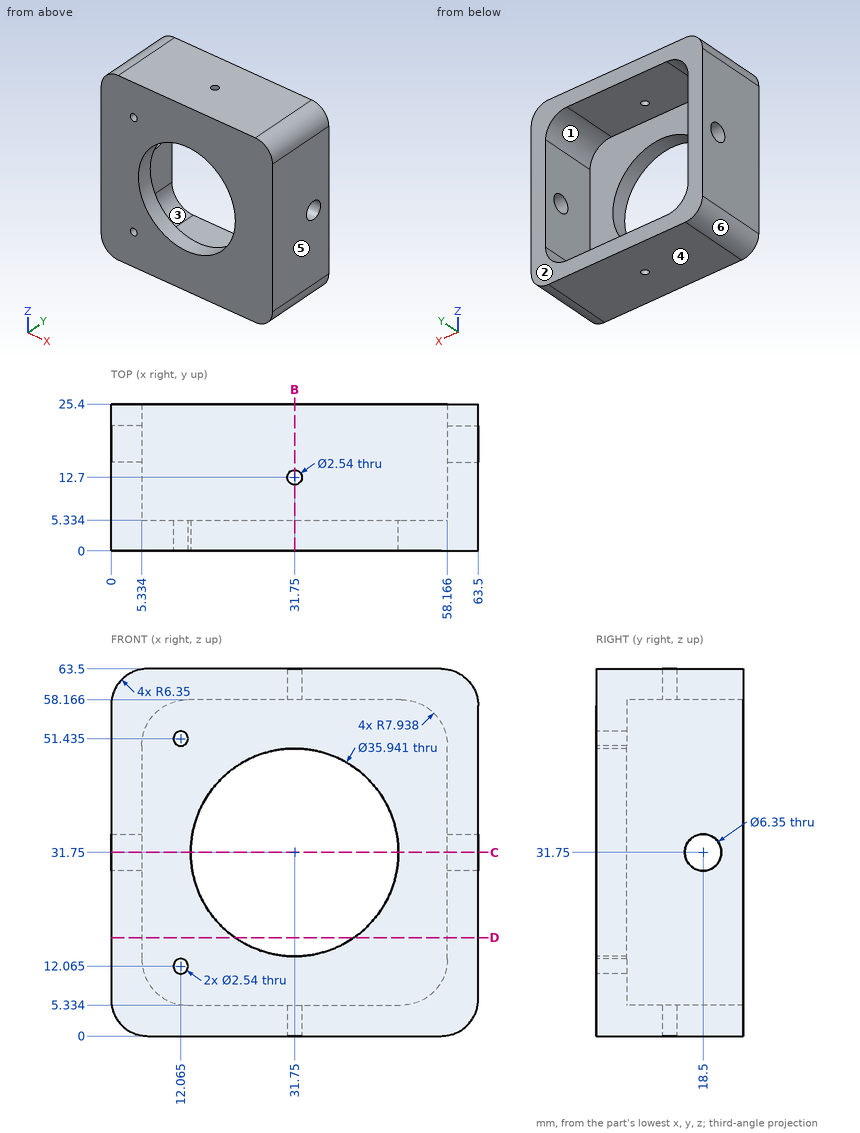
Here's the drawing with two shaded views (mm, measured from the low corner). I have some questions. A direction names the side the tool comes from. Coordinates: 2 decimals unless noted, no trailing zeros. Write each loop counter-clockwise with the first axis right and the second up, starting at its lowest first coordinate (ties: lowest second). Pieces come first, ordered by that corner, then holes. Notation, with made-up numbers: M 19.25,76 L 62.25,76 A10 ccw 62.25,80 Z; hole C 53,88.25 d10. An arc over 180 degrees is marked long. Use one line per item in the form item = value.
Q1. If we section it at D-D (z = 17): Write out the boundary of the cut face in (x, y) (1 decimal), then the cut area to 3 significant figures.
Model answer:
outline = M 0,0 L 21.5,0 L 21.5,5.3 L 5.3,5.3 L 5.3,25.4 L 0,25.4 Z; M 42,0 L 63.5,0 L 63.5,25.4 L 58.2,25.4 L 58.2,5.3 L 42,5.3 Z
area = 443 mm^2
Q2. If we section it at C-C (z = 31.75): Write out the boundary of the cut face in (x, y) (1 decimal).
Model answer:
outline = M 0,0 L 13.8,0 L 13.8,5.3 L 5.3,5.3 L 5.3,15.3 L 0,15.3 Z; M 0,21.7 L 5.3,21.7 L 5.3,25.4 L 0,25.4 Z; M 49.7,0 L 63.5,0 L 63.5,15.3 L 58.2,15.3 L 58.2,5.3 L 49.7,5.3 Z; M 58.2,21.7 L 63.5,21.7 L 63.5,25.4 L 58.2,25.4 Z
Q3. I need wall thicknesses on line 1 along Z through (x, y) = (19, 12.25) (1 decimal); line 2 along Y through (x, z) = (31.75, 3.25). Which ranges of each line are inside material? Lowest first, please. Write a range as from..to.
Model answer:
line_1 = 0..5.3, 58.2..63.5
line_2 = 0..11.43, 13.97..25.4
Q4. For the marked faces 1 and 2, which set-ups out of +Z, -Z, +X, -X, +Y, -Y let a thin tool reach every point of the face, with its end or its side?
Model answer:
face_1 = +Y
face_2 = +Z, -Z, +X, -X, +Y
Q5. If we section it at B-B (x = 31.75): Write out the boundary of the cut face in (y, z) (1 decimal).
Model answer:
outline = M 0,0 L 11.4,0 L 11.4,5.3 L 5.3,5.3 L 5.3,13.8 L 0,13.8 Z; M 0,49.7 L 5.3,49.7 L 5.3,58.2 L 11.4,58.2 L 11.4,63.5 L 0,63.5 Z; M 14,0 L 25.4,0 L 25.4,5.3 L 14,5.3 Z; M 14,58.2 L 25.4,58.2 L 25.4,63.5 L 14,63.5 Z
Q6. For P1, Ø4, axis at x = 42, z = 19, coming from the +Y side, with a flat end and sliding along its axis, tell me the tip position at first contact or that it passes through.
Model answer:
P1 = 5.33
Q7. We'd pull the mould along X, two halves only. Please class the marked faces 3, 4, 5 and 6: +X half, -X half, draft (parallel to the pull), parting line (faces both ways), or undercut.
Model answer:
face_3 = undercut
face_4 = draft
face_5 = +X half
face_6 = -X half
